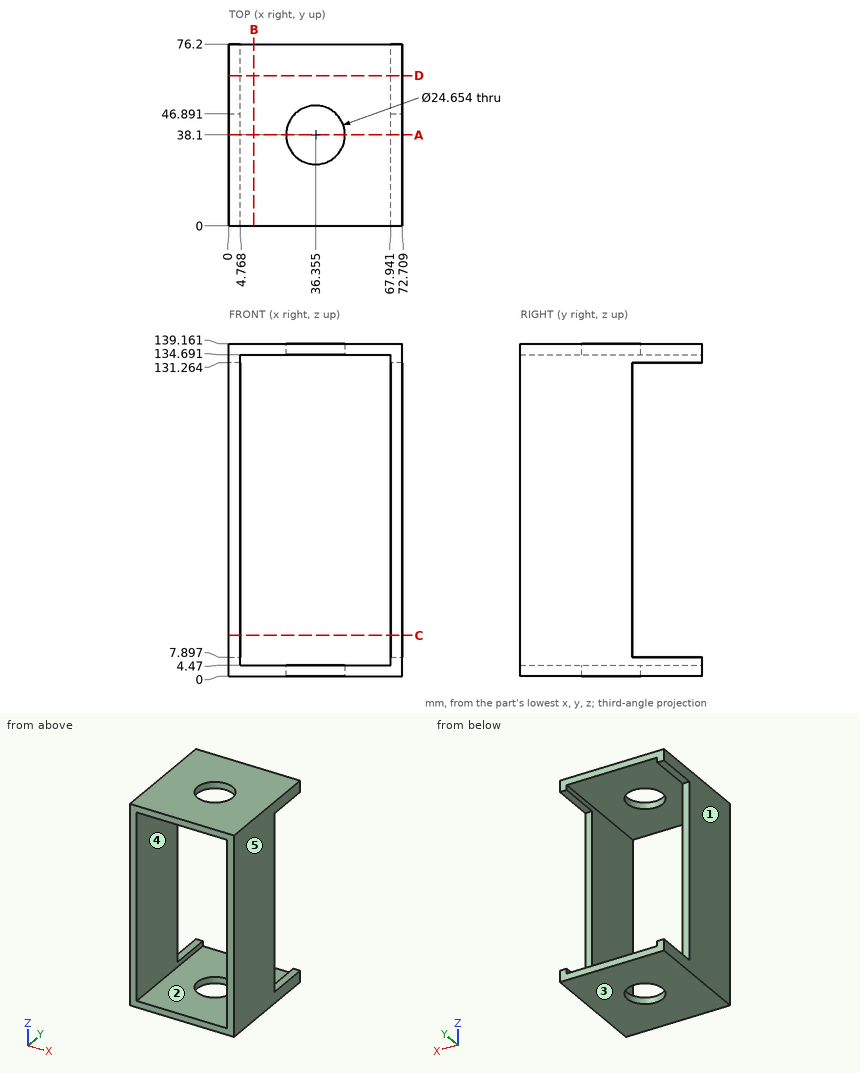
Here's the drawing with two shaded views (mm, measured from the low corner). I have some questions. A direction names the side the tool comes from. Give positions to 0.01 mm unless a question says otherwise; leave off trailing zeros. Order: outer loops, then holes, each group sorted by start corner. A loop starts at its lowest first (then second) coordinate and runs counter-clockwise, first axis right, second up. Notation, with made-up numbers: (11, -13.5) - (53, -13.5) arc R24 cw to (53, 4.5) - close; hole circle Ø10 at (42.5, 3). An arc over 180 degrees is marked (long way). Write each question's results on one line, items separated by ' | '.
1) Please list where these lines run through material, in increasing order: line 1 along X through (y, z) = (38, 3); line 2 along Z through (x, y) = (65.5, 19.5); line 3 along X through (y, z) = (34.5, 55). Write a range as [from, to].
Final values:
line 1: x = [0, 24.03], [48.68, 72.71] | line 2: z = [0, 4.47], [134.69, 139.16] | line 3: x = [0, 4.77], [67.94, 72.71]
2) Suppose I cut it at B-B, the plane x = 10.5. Write out the boundary of the cut face in (y, z), then the cut area to 3 significant figures.
Final values:
outline: (0, 0) - (76.2, 0) - (76.2, 4.47) - (0, 4.47) - close; (0, 134.69) - (76.2, 134.69) - (76.2, 139.16) - (0, 139.16) - close | area: 681 mm^2
3) If we mould it in two halves opening along X, with no side actions, what happens to the marked faces 3, 4 and 5? For each: pulls with the +X half, pulls with the -X half, needs draft (parallel to the pull), parting line crosses it, or undercut.
Final values:
face 3: needs draft | face 4: undercut | face 5: pulls with the +X half
4) Suppose I cut it at C-C, the plane z = 17. Write out the boundary of the cut face in (x, y).
Final values:
outline: (0, 0) - (4.77, 0) - (4.77, 46.89) - (0, 46.89) - close; (67.94, 0) - (72.71, 0) - (72.71, 46.89) - (67.94, 46.89) - close
5) Suppose I cut it at D-D, the plane y = 63. Write out the boundary of the cut face in (x, z).
Final values:
outline: (0, 0) - (72.71, 0) - (72.71, 7.9) - (67.94, 7.9) - (67.94, 4.47) - (4.77, 4.47) - (4.77, 7.9) - (0, 7.9) - close; (0, 131.26) - (4.77, 131.26) - (4.77, 134.69) - (67.94, 134.69) - (67.94, 131.26) - (72.71, 131.26) - (72.71, 139.16) - (0, 139.16) - close
6) Suppose I cut it at A-A, the plane y = 38.1. Write out the boundary of the cut face in (x, z).
Final values:
outline: (0, 0) - (24.03, 0) - (24.03, 4.47) - (4.77, 4.47) - (4.77, 134.69) - (24.03, 134.69) - (24.03, 139.16) - (0, 139.16) - close; (48.68, 0) - (72.71, 0) - (72.71, 139.16) - (48.68, 139.16) - (48.68, 134.69) - (67.94, 134.69) - (67.94, 4.47) - (48.68, 4.47) - close
7) I'm going to push flat-ended pins straight in: pin 1 Ø19.5 at (x, y) = (36.35, 38.1) entering from -Z; pin 2 Ø5 at (x, y) = (3, 67) entering from -Z; pin 3 Ø2.5 at (x, z) = (71.5, 87.5) entering from +Y. Where does each tip first touch, or does it pass through?
Final values:
pin 1: passes through | pin 2: stops at z = 0 | pin 3: stops at y = 46.89
8) On a 3-axis mill with a long thin cutter (end or side, diameter ignored), from which of +Z, -Z, +X, -X, +Y, -Y can I reach the whole of each face in a straight line? I mean the marked faces 1 and 2. Say none if no direction works.
Final values:
face 1: +Z, -Z, -X, +Y, -Y | face 2: +Y, -Y
